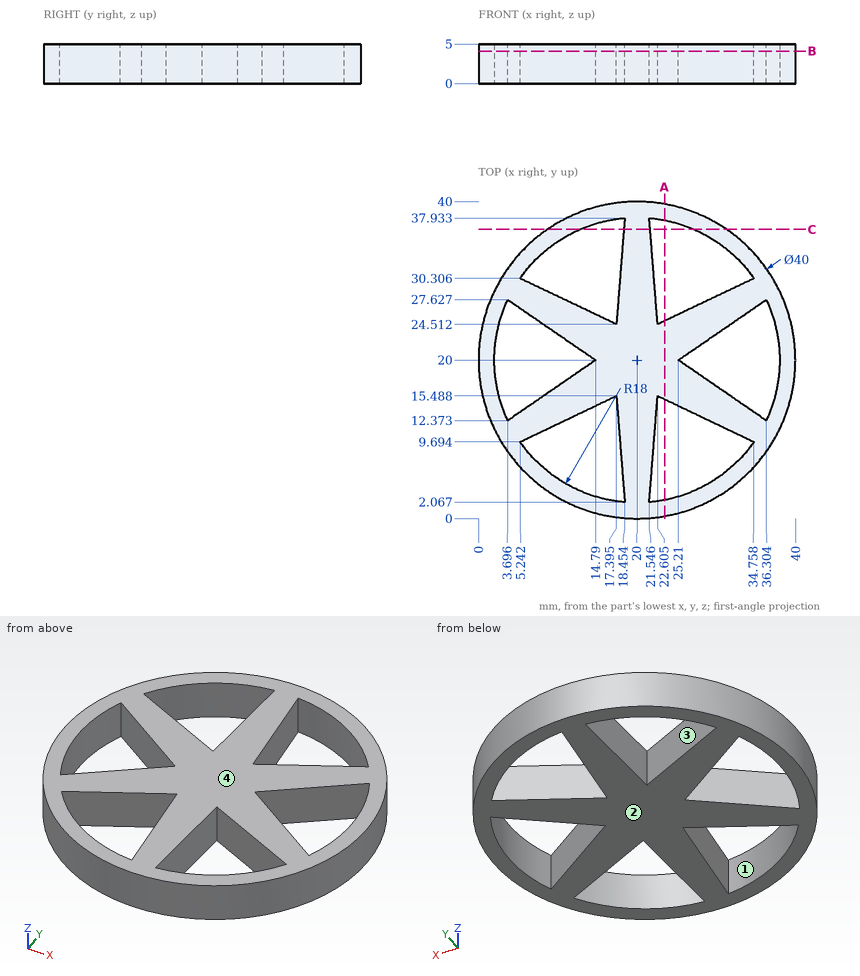
Geometry: see drawing. Coordinates: mm, zero at the bounding-box minimum. A direction names the side the tool comes from. Round coordinates to 2 decimals unless told otherwise and drop trailing zeros. Write each loop counter-clockwise with the first axis right and the second up, starting at its lowest first coordinate (ties: lowest second). Pieces come first, ordered by that corner, then holes. Notation, with made-up numbers: (-40, 19.25) -> (-32, 19.25) arc R30 ccw to (-32, 44.25) -> close; hole circle Ø6 at (29, -15.75). An arc over 180 degrees is marked (long way). Answer as CSV lines item,"result".
1. Section A-A (x = 23.5). Return the cut outline in (y, z).
Geometry says:
outline,"(0.31, 0) -> (2.34, 0) -> (2.34, 5) -> (0.31, 5) -> close; (15.06, 0) -> (24.94, 0) -> (24.94, 5) -> (15.06, 5) -> close; (37.66, 0) -> (39.69, 0) -> (39.69, 5) -> (37.66, 5) -> close"
2. Contact query for flat-ended pins moving along their axis: P1, Ø3, axis at y = 11.5, z = 4, coming from the +X side (1 decimal); P2, Ø1, axis at y = 23.5, z = 0.5, coming from the +X side. Output: stop coordinate, or through.
Geometry says:
P1,"stops at x = 38.7"
P2,"stops at x = 39.77"
3. Reachability of the marked faces 3 and 4 from +Z, -Z, +X, -X, +Y, -Y: full face, straight path, thin tool, end or side. Return the list, or none.
Geometry says:
face 3,"+Z, -Z"
face 4,"+Z, +X, -X, +Y, -Y"
4. Section C-C (y = 36.5). Return the cut outline in (x, z).
Geometry says:
outline,"(8.7, 0) -> (12.81, 0) -> (12.81, 5) -> (8.7, 5) -> close; (18.34, 0) -> (21.66, 0) -> (21.66, 5) -> (18.34, 5) -> close; (27.19, 0) -> (31.3, 0) -> (31.3, 5) -> (27.19, 5) -> close"
5. Mould query, pull axis Y, two halves, no side actions, for the marked faces 1 and 2. Classes: +Y half, -Y half, draft (parallel to the pull), parting line (faces both ways), or undercut.
Geometry says:
face 1,"undercut"
face 2,"draft"
6. Ray query, L1, parallel to X at y = 30.5, z = 3.3 (1 decimal); L2, parallel to X at y = 14, z = 1.6 (1 decimal); L3, parallel to Y at x = 6, z = 3.15 (1 decimal). Return the intervals inside material, ascending. Write a range as [from, to].
Geometry says:
L1,"x = [3, 5.4], [17.9, 22.1], [34.6, 37]"
L2,"x = [0.9, 3], [6.1, 14.3], [17.5, 22.5], [25.7, 33.9], [37, 39.1]"
L3,"y = [5.7, 8.7], [10.1, 14], [26, 29.9], [31.3, 34.3]"
7. Section B-B (z = 4.1). Return the cut outline in (x, y) (1 decimal).
Geometry says:
outline,"circle Ø40 at (20, 20); hole (3.7, 12.4) -> (14.8, 20) -> (3.7, 27.6) arc R18 ccw to start; hole (5.2, 9.7) arc R18 ccw to (18.5, 2.1) -> (17.4, 15.5) -> close; hole (5.2, 30.3) -> (17.4, 24.5) -> (18.5, 37.9) arc R18 ccw to start; hole (21.5, 2.1) arc R18 ccw to (34.8, 9.7) -> (22.6, 15.5) -> close; hole (21.5, 37.9) -> (22.6, 24.5) -> (34.8, 30.3) arc R18 ccw to start; hole (25.2, 20) -> (36.3, 12.4) arc R18 ccw to (36.3, 27.6) -> close"
